from build123d import *

# Parameters (mm, degrees)
SKETCH1_R                   = 9.525
BOSS_EXTRUDE1_DEPTH         = 495.3
F_1_4_20_TAPPED_HOLE1_D     = 5.1054
F_1_4_20_TAPPED_HOLE1_DEPTH = 16.51
F_1_4_20_TAPPED_HOLE1_TIP   = 1.533816902
F_1_4_20_TAPPED_HOLE2_D     = 5.1054
F_1_4_20_TAPPED_HOLE2_DEPTH = 16.51
F_1_4_20_TAPPED_HOLE2_TIP   = 1.533816902


with BuildPart() as part:
    # Sketch1 → Boss-Extrude1 (new body)
    with BuildSketch(Plane(origin=(0, 0, 0), x_dir=(0, 0, -1), z_dir=(1, 0, 0))):
        Circle(SKETCH1_R)
    extrude(amount=-BOSS_EXTRUDE1_DEPTH)

    # 1/4-20 Tapped Hole1
    with Locations(Plane(origin=(0, 0, 0), x_dir=(0, 0, -1), z_dir=(1, 0, 0))):
        with Locations((0, 0)):
            Hole(F_1_4_20_TAPPED_HOLE1_D / 2, depth=F_1_4_20_TAPPED_HOLE1_DEPTH)
            with Locations((0, 0, -(F_1_4_20_TAPPED_HOLE1_DEPTH + F_1_4_20_TAPPED_HOLE1_TIP / 2))):  # 118° drill point
                Cone(0, F_1_4_20_TAPPED_HOLE1_D / 2, F_1_4_20_TAPPED_HOLE1_TIP, mode=Mode.SUBTRACT)

    # 1/4-20 Tapped Hole2
    with Locations(Plane.ZY.offset(495.3)):
        with Locations((0, 0)):
            Hole(F_1_4_20_TAPPED_HOLE2_D / 2, depth=F_1_4_20_TAPPED_HOLE2_DEPTH)
            with Locations((0, 0, -(F_1_4_20_TAPPED_HOLE2_DEPTH + F_1_4_20_TAPPED_HOLE2_TIP / 2))):  # 118° drill point
                Cone(0, F_1_4_20_TAPPED_HOLE2_D / 2, F_1_4_20_TAPPED_HOLE2_TIP, mode=Mode.SUBTRACT)


solid = part.part
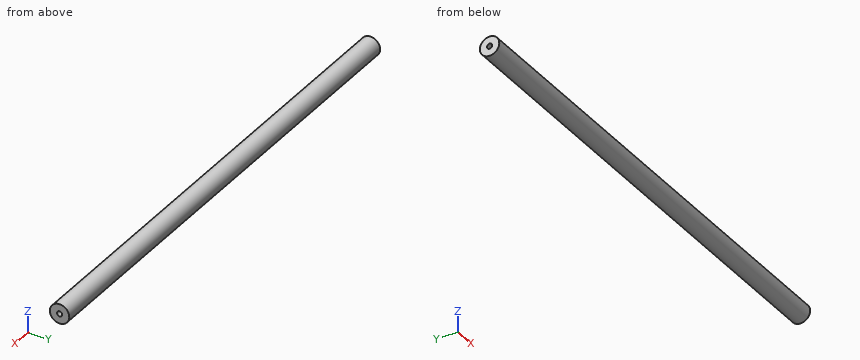
Check sheet for the modelled part. Datum: model origin and axes. Units: mm. Coordinates: 2 decimals unless noted, no trailing zeros. Write each loop counter-clockwise with the first axis right and the second up, starting at its lowest first coordinate (ties: lowest second). Pieces come first, ordered by that corner, then holes.
Item 1: Scan lines: probe 1 along Y at (x, z) = (-11, 0) (3 decimals); probe 2 along Z at (x, y) = (-342, 0.5). Record each from-to range of solid material in increasing order.
Numbers:
probe 1: y = -9.525 to -2.553, 2.553 to 9.525
probe 2: z = -9.51 to 9.51
Item 2: Depth check by flat-ended pin: pin 1 Ø1 at (x, z) = (-256.5, 5.5) entering from -Y; pin 2 Ø1.5 at (x, y) = (-187, -4) entering from +Z; pin 3 Ø4 at (x, z) = (-232.5, 7.5) entering from +Y. Enter the tip coordinate at first touch or a pass-through.
Numbers:
pin 1: stops at y = -8.11
pin 2: stops at z = 8.95
pin 3: stops at y = 7.78
Item 3: Cross-section at A-A on x = -113.5. Record the boundary of the cut face in (y, z) (3 decimals).
Numbers:
outline: circle Ø19.05 at (0, 0)
Item 4: Cross-section at C-C on z = 6.5. Record the boundary of the cut face in (x, y).
Numbers:
outline: (-495.3, -6.96) - (0, -6.96) - (0, 6.96) - (-495.3, 6.96) - close
Item 5: Cross-section at B-B on y = 6.25. Record the boundary of the cut face in (x, z).
Numbers:
outline: (-495.3, -7.19) - (0, -7.19) - (0, 7.19) - (-495.3, 7.19) - close
